Here's how the part is built. I have some questions about the finished solid (model axes, mm). Face numbers are marked on the shaded views. A direction names the side the tool comes from. Round coordinates to 2 decimals unless told otherwise and drop trailing zeros. Order: outer loops, then holes, each group sorted by start corner. A loop starts at its lowest first (then second) coordinate and runs counter-clockwise, first axis right, second up. Notation, with made-up numbers: M 67.5,87 L 76.5,87 A25 ccw 76.5,126 Z; hole C 29,72.5 d2. An arc over 180 degrees is marked long. Write item = value, one per line. Start each with the question number.
Item 1: I want a section at C-C, the plane y = 0.5. List the corners of the cut face in (x, z) for me.
Item 2: I want a section at B-B, the plane x = 10.5. List the corners of the cut face in (y, z) for me, plus the area to 3 significant figures.
Item 3: For the marked faces 1 and 2, which set-ups out of +Z, -Z, +X, -X, +Y, -Y let a thin tool reach every point of the face, with its end or its side?
Item 4: I want a section at D-D, the plane y = 1.3. List the corners of the cut face in (x, z) for me, plus the area to 3 significant figures.
Item 5: I'm going to push a flat-ended pin straight in: P1, Ø1, axis at x = 16.5, z = 5, coming from the +Y side. Where does the tip first touch, or does it pass through?
Item 6: Please list where these lines run through material, in increasing order: L1, parallel to Y at x = 8.75, z = 12.5; L2, parallel to Z at x = 8, y = 0.5 (3 decimals); L3, parallel to X at y = 0.15, z = 11.
Item 7: I want a section at A-A, the plane z = 1. List the corners of the cut face in (x, y) for me.
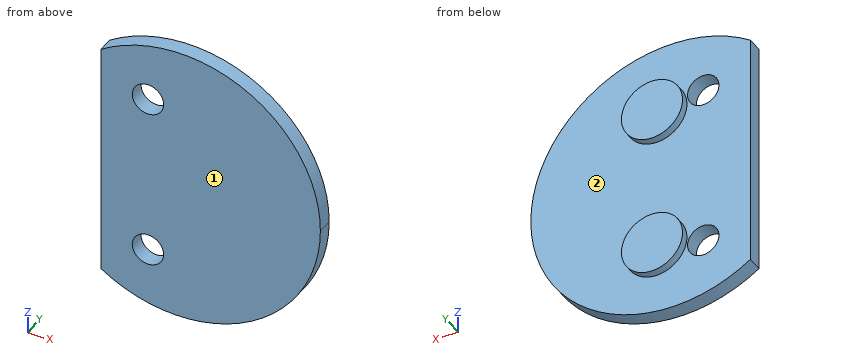
```python
from build123d import *

# Parameters (mm, degrees)
RESSALTO_EXTRUS_O2_DEPTH   = 1.5
ESBO_O5_R                  = 15.72745668
ESBO_O5_R_2                = 1.945049623
CORTE_EXTRUS_O1_DEPTH      = 0.5
CORTE_EXTRUS_O2_DEPTH      = 24.840358488
CORTE_EXTRUS_O2_DEPTH_BACK = 24.840358488
ESBO_O7_R                  = 1


with BuildPart() as part:
    # Esboço4 → Ressalto-extrusão2 (new body)
    with BuildSketch(Plane(origin=(0, 0, 0), x_dir=(1, 0, 0), z_dir=(0, 1, 0))):
        with BuildLine():
            ThreePointArc((18.945063587, -5.437702675), (14.200975083, 2.492443436), (4.970126401, 2.062297325))
            Line((4.970126401, 2.062297325), (4.970126401, -12.937702675))
            ThreePointArc((4.970126401, -12.937702675), (14.200975083, -13.367848785), (18.945063587, -5.437702675))
        make_face()
    extrude(amount=RESSALTO_EXTRUS_O2_DEPTH)

    # Esboço5 → Corte-extrusão1 (cut)
    with BuildSketch(Plane(origin=(0, 1.5, 0), x_dir=(1, 0, 0), z_dir=(0, 1, 0))):
        with Locations((8.279998828, -5.161239755)):
            Circle(ESBO_O5_R)
        with Locations(Location((10.953382727, -0.888525014, 0), (0, 0, 270))):
            Circle(ESBO_O5_R_2, mode=Mode.SUBTRACT)
        with Locations(Location((10.953382727, -9.986880335, 0), (0, 0, 270))):
            Circle(ESBO_O5_R_2, mode=Mode.SUBTRACT)
    extrude(amount=-CORTE_EXTRUS_O1_DEPTH, mode=Mode.SUBTRACT)

    # Esboço7 → Corte-extrusão2 (cut, two sides: drawn at the far end of the back side and taken through both)
    with BuildSketch(Plane(origin=(0, 1, 0), x_dir=(1, 0, 0), z_dir=(0, 1, 0)).offset(-CORTE_EXTRUS_O2_DEPTH_BACK)):
        with Locations(Location((7.970126401, -10.572389641, 0), (0, 0, 270))):
            Circle(ESBO_O7_R)
        with Locations(Location((7.970126401, -0.303015709, 0), (0, 0, 270))):
            Circle(ESBO_O7_R)
    extrude(amount=CORTE_EXTRUS_O2_DEPTH + CORTE_EXTRUS_O2_DEPTH_BACK, mode=Mode.SUBTRACT)


solid = part.part
```
Filled in:
q1.outline = M 4.97,-2.06 A9 ccw long 4.97,12.94 Z; hole C 7.97,0.3 d2; hole C 7.97,10.57 d2
q2.outline = M 0,-3.55 L 1,-3.55 L 1,-1 L 1.5,-1 L 1.5,2.78 L 1,2.78 L 1,8.1 L 1.5,8.1 L 1.5,11.88 L 1,11.88 L 1,14.42 L 0,14.42 Z
q2.area = 21.7 mm^2
q3.face_1 = +Z, -Z, +X, -X, -Y
q3.face_2 = +Y
q4.outline = C 10.95,0.89 d3.89; C 10.95,9.99 d3.89
q4.area = 23.8 mm^2
q5.P1 = 1
q6.L1 = 0 to 1
q6.L2 = -3.35 to -0.697, 1.303 to 9.573, 11.572 to 14.225
q6.L3 = 4.97 to 7.07, 8.87 to 17.02
q7.outline = M 4.97,0 L 7.25,0 L 7.25,1 L 4.97,1 Z; M 8.69,0 L 17.77,0 L 17.77,1 L 12.9,1 L 12.9,1.5 L 9.01,1.5 L 9.01,1 L 8.69,1 Z
